Autodesk Inventor part; units mm, degrees
ref_plane "YZ Plane" through (0, 0, 0) normal (1, 0, 0) x (0, 1, 0)
ref_plane "XZ Plane" through (0, 0, 0) normal (0, 1, 0) x (-1, 0, 0)
ref_plane "XY Plane" through (0, 0, 0) normal (0, 0, 1) x (1, 0, 0)
sketch "Esquisse1" plane through (0, 0, 0) normal (0, 0, 1) x (1, 0, 0)
  circle A0 centre (0, 0) radius 40
  circle A1 centre (0, 0) radius 12
  line L0 (0, 0) -> (-13.5, 0) construction
  line L1 (-13.5, 0) -> (-13.5, 6.5) construction
  line L2 (-13.5, 6.5) -> (-13.5, 14.5) construction
  line L3 (-13.5, 14.5) -> (-13.5, 22.5) construction
  line L4 (-13.5, 22.5) -> (-13.5, 30.5) construction
  line L5 (0, 0) -> (0, 36) construction
  line L6 (0, 36) -> (-8, 36) construction
  circle A2 centre (-13.5, 6.5) radius 1
  circle A3 centre (-13.5, 14.5) radius 1
  circle A4 centre (-13.5, 22.5) radius 1
  circle A5 centre (-13.5, 30.5) radius 1
  circle A6 centre (-8, 36) radius 1
  circle A7 centre (13.5, 6.5) radius 1
  circle A8 centre (13.5, 14.5) radius 1
  circle A9 centre (13.5, 22.5) radius 1
  circle A10 centre (13.5, 30.5) radius 1
  circle A11 centre (8, 36) radius 1
  line L7 (0, 0) -> (40, 0) construction
  line L8 (12, 0) -> (40, 0) construction
  circle A12 centre (26, 0) radius 2
  circle A13 centre (0, 26) radius 2
  circle A14 centre (-26, 0) radius 2
  circle A15 centre (0, -26) radius 2
  line L9 (0, 0) -> (0, -26) construction
  dimension "d0" = 80
  dimension "d1" = 24
  dimension "d2" = 13.5
  dimension "d3" = 6.5
  dimension "d4" = 8
  dimension "d5" = 8
  dimension "d6" = 8
  dimension "d7" = 36
  dimension "d8" = 8
  dimension "d9" = 2
  dimension "d25" = 4
  dimension "d28" = 360
  dimension "d39" = 26
extrude "Extrusion3" add sketch "Esquisse1" along normal blind 9
sketch "Esquisse5" plane through (0, 0, 9) normal (0, 0, 1) x (1, 0, 0)
  circle A0 centre (0, 0) radius 12
  circle A1 centre (0, -26) radius 2
  circle A2 centre (-26, 0) radius 2
  circle A3 centre (0, 26) radius 2
  circle A4 centre (26, 0) radius 2
  circle A5 centre (0, 0) radius 40
  line L0 (0, 0) -> (40, 0) construction
  line L1 (29.5, 2.0207) -> (29.5, -2.0207)
  line L2 (29.5, -2.0207) -> (26, -4.0415)
  line L3 (26, -4.0415) -> (22.5, -2.0207)
  line L4 (22.5, -2.0207) -> (22.5, 2.0207)
  line L5 (22.5, 2.0207) -> (26, 4.0415)
  line L6 (26, 4.0415) -> (29.5, 2.0207)
  line L7 (22.5, 2.0207) -> (29.5, 2.0207) construction
  line L8 (-2.0207, 29.5) -> (2.0207, 29.5)
  line L9 (2.0207, 29.5) -> (4.0415, 26)
  line L10 (4.0415, 26) -> (2.0207, 22.5)
  line L11 (2.0207, 22.5) -> (-2.0207, 22.5)
  line L12 (-2.0207, 22.5) -> (-4.0415, 26)
  line L13 (-4.0415, 26) -> (-2.0207, 29.5)
  line L14 (-29.5, -2.0207) -> (-29.5, 2.0207)
  line L15 (-29.5, 2.0207) -> (-26, 4.0415)
  line L16 (-26, 4.0415) -> (-22.5, 2.0207)
  line L17 (-22.5, 2.0207) -> (-22.5, -2.0207)
  line L18 (-22.5, -2.0207) -> (-26, -4.0415)
  line L19 (-26, -4.0415) -> (-29.5, -2.0207)
  line L20 (2.0207, -29.5) -> (-2.0207, -29.5)
  line L21 (-2.0207, -29.5) -> (-4.0415, -26)
  line L22 (-4.0415, -26) -> (-2.0207, -22.5)
  line L23 (-2.0207, -22.5) -> (2.0207, -22.5)
  line L24 (2.0207, -22.5) -> (4.0415, -26)
  line L25 (4.0415, -26) -> (2.0207, -29.5)
  dimension "d50" = 7
  dimension "d53" = 360
extrude "Extrusion7" cut sketch "Esquisse5" against normal blind 3 contours L1 L2 L3 L4 L5 L6 | L8 L9 L10 L11 L12 L13 | L14 L15 L16 L17 L18 L19 | L20 L21 L22 L23 L24 L25
properties part number "bowl_ax12_support_v2"
Check sheet for the modelled part. Datum: model origin and axes. Units: mm. A direction names the side the tool comes from. Round coordinates to 2 decimals unless told otherwise and drop trailing zeros. Order: outer loops, then holes, each group sorted by start corner. A loop starts at its lowest first (then second) coordinate and runs counter-clockwise, first axis right, second up. Notation, with made-up numbers: (45.5, 35.5) -> (92.5, 35.5) arc R7 cw to (92.5, 44.5) -> close; hole circle Ø11 at (67.5, 57.25). An arc over 180 degrees is marked (long way). One line per item, written item: value. Start each with the question number.
Q1. Cross-section at B-B (x = 8). Record the boundary of the cut face in (y, z).
Q2. Thickness scan on line 1 (Y direction, x = 0, z = 4.6); line 2 (Y direction, x = 0, z = 7.25); line 3 (Y direction, x = 13.5, z = 3.75). Record the ranges inside material, lowest first.
Q3. Set-up check for faces 1 (the face through (3, -24.2, 7.5)), 2 (the face through (-12.546, 6.2, 4.437)): record each of +Z, -Z, +X, -X, +Y, -Y from which the full face is reachable in a straight line by a thin tool's end or side.
Q4. Mould release check, pull along X, two halves, no side actions. Record for faces 3 (the face through (24.2, 3, 7.5)), 4 (the face through (2, 28, 6)), 5 (the face through (-9.4, -8.3, 9)), 6 (the face through (-8.67, 39.05, 4.44)): pulls with the +X half, pulls with the -X half, needs draft (parallel to the pull), parting line crosses it, or undercut.
Q5. Cross-section at A-A (z = 3.5). Give the number of separate pieces and of enclosed holes in the cut face, and give its area (3 significant figures).
Q6. Cross-section at D-D (x = -13.5). Record the boundary of the cut face in (y, z), and give its area (3 significant figures).
Q7. Cross-section at C-C (y = 30.5). Record the boundary of the cut face in (x, z), and give its area (3 significant figures).
Q8. Gauge pin test, flat ends, axial feed: pin 1 Ø4 at (y, z) = (-18.5, 2) entering from +X; pin 2 Ø3 at (x, y) = (-8, 36) entering from -Z; pin 3 Ø2 at (x, y) = (1.5, -27) entering from +Z; pin 4 Ø2 at (x, z) = (31.5, 5) entering from +Y. Record the tip position at first contact, or that the pin passes through.
Completed:
1. outline: (-39.19, 0) -> (-8.94, 0) -> (-8.94, 9) -> (-39.19, 9) -> close; (8.94, 0) -> (35, 0) -> (35, 9) -> (8.94, 9) -> close; (37, 0) -> (39.19, 0) -> (39.19, 9) -> (37, 9) -> close
2. line 1: y = -40 to -28, -24 to -12, 12 to 24, 28 to 40
2. line 2: y = -40 to -29.5, -22.5 to -12, 12 to 22.5, 29.5 to 40
2. line 3: y = -37.65 to 5.5, 7.5 to 13.5, 15.5 to 21.5, 23.5 to 29.5, 31.5 to 37.65
3. face 1: +Z
3. face 2: +Z, -Z
4. face 3: undercut
4. face 4: undercut
4. face 5: needs draft
4. face 6: parting line crosses it
5. separate pieces: 1
5. enclosed holes: 15
5. area: 4,490 mm²
6. outline: (-37.65, 0) -> (5.5, 0) -> (5.5, 9) -> (-37.65, 9) -> close; (7.5, 0) -> (13.5, 0) -> (13.5, 9) -> (7.5, 9) -> close; (15.5, 0) -> (21.5, 0) -> (21.5, 9) -> (15.5, 9) -> close; (23.5, 0) -> (29.5, 0) -> (29.5, 9) -> (23.5, 9) -> close; (31.5, 0) -> (37.65, 0) -> (37.65, 9) -> (31.5, 9) -> close
6. area: 606 mm²
7. outline: (-25.88, 0) -> (-14.5, 0) -> (-14.5, 9) -> (-25.88, 9) -> close; (-12.5, 0) -> (12.5, 0) -> (12.5, 9) -> (-12.5, 9) -> close; (14.5, 0) -> (25.88, 0) -> (25.88, 9) -> (14.5, 9) -> close
7. area: 430 mm²
8. pin 1: stops at x = 36.44
8. pin 2: stops at z = 0
8. pin 3: stops at z = 6
8. pin 4: stops at y = 25.88
